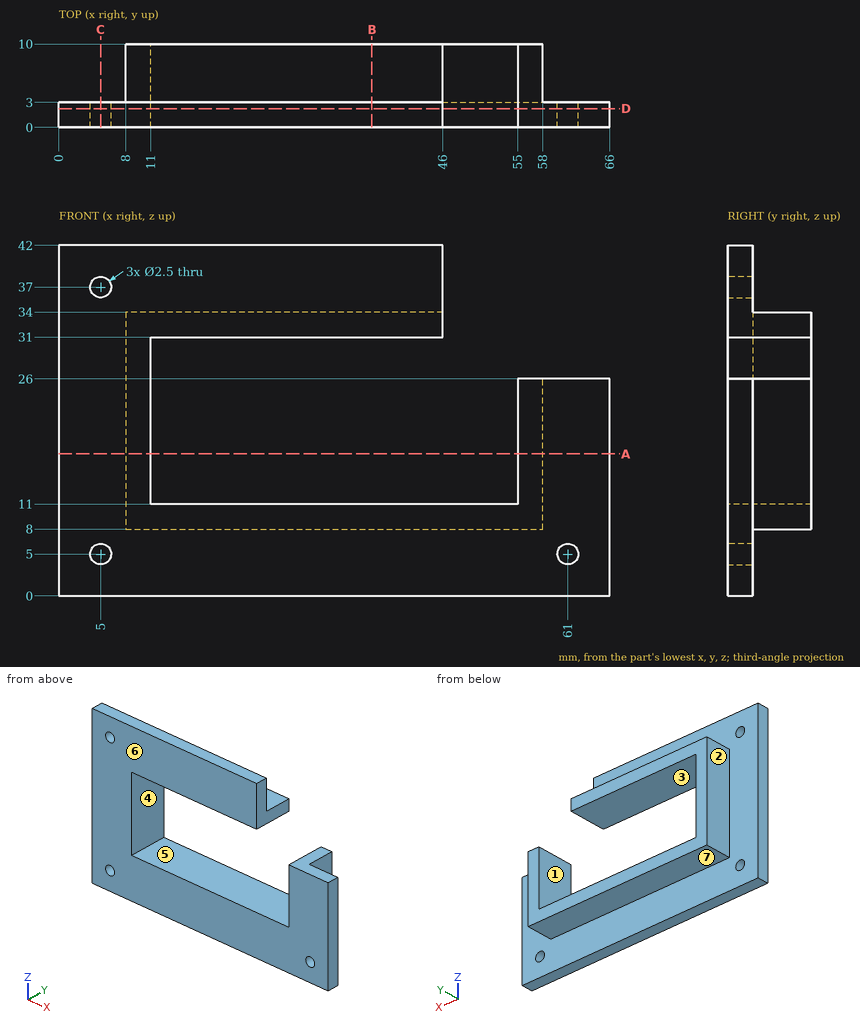
Job drawing, mm, ordinate dimensions from the low corner. One solid piece. A direction names the side the tool comes from. Round coordinates to 2 decimals unless told otherwise and drop trailing zeros. Loops run counter-clockwise (first coordinate to the right, second up) from the corner with the lowest first, then second, coordinate; pieces in that order, holes last. Notation, with made-up numbers: (46, 80) -> (105, 80) arc R28 cw to (105, 103) -> close; hole circle Ø7 at (-40, -12). An arc over 180 degrees is marked (long way). One line per item, written item: value. Start each with the question number.
Q1. Probe line 1 along X through (y, z) = (1.95, 5); line 2 along Z through (x, y) = (36.5, 2); line 3 along X through (y, z) = (1.65, 37). List the from-to ranges inside material, lowest first.
Q2. Cut at C-C on x = 5. List the corners of the cut face in (y, z).
Q3. 3-axis set-ups, long thin cutter, end or side, ignore diameter. For the marked faces 1, 2, 3 and 4: which of +Z, -Z, +X, -X, +Y, -Y reach the whole face in a straight line?
Q4. Cut at D-D on y = 2.25. List the corners of the cut face in (x, z).
Q5. Drop flat-ended pins along their axis: pin 1 Ø6 at (x, z) = (32.5, 28.5) entering from -Y; pin 2 Ø1 at (y, z) = (8.5, 26) entering from +X; pin 3 Ø4 at (x, z) = (5, 5) entering from +Y; pin 4 Ø3 at (x, y) = (51, 1) entering from +Z. Give the stop position or say it passes through.
Q6. Two-plate mould, pull along Z, no slides. Class the marked faces 5, 6 and 7: released by +Z, released by -Z, zero draft, split by the parting line, or undercut.
Q7. Cut at A-A on z = 17. List the corners of the cut face in (x, y), plus the area to 3 significant figures.
Q8. Cut at B-B on x = 37.5. List the corners of the cut face in (y, z), plus the area to 3 significant figures.
Computed:
1. line 1: 0 to 3.75, 6.25 to 59.75, 62.25 to 66
1. line 2: 0 to 11, 31 to 42
1. line 3: 0 to 3.75, 6.25 to 46
2. outline: (0, 0) -> (3, 0) -> (3, 3.75) -> (0, 3.75) -> close; (0, 6.25) -> (3, 6.25) -> (3, 35.75) -> (0, 35.75) -> close; (0, 38.25) -> (3, 38.25) -> (3, 42) -> (0, 42) -> close
3. face 1: +Z, +Y, -Y
3. face 2: +Z, -Z, -X, +Y
3. face 3: +X, +Y, -Y
3. face 4: +Y, -Y
4. outline: (0, 0) -> (66, 0) -> (66, 26) -> (55, 26) -> (55, 11) -> (11, 11) -> (11, 31) -> (46, 31) -> (46, 42) -> (0, 42) -> close; hole circle Ø2.5 at (5, 5); hole circle Ø2.5 at (5, 37); hole circle Ø2.5 at (61, 5)
5. pin 1: y = 0
5. pin 2: x = 58
5. pin 3: y = 3
5. pin 4: z = 11
6. face 5: undercut
6. face 6: zero draft
6. face 7: released by -Z
7. outline: (0, 0) -> (11, 0) -> (11, 10) -> (8, 10) -> (8, 3) -> (0, 3) -> close; (55, 0) -> (66, 0) -> (66, 3) -> (58, 3) -> (58, 10) -> (55, 10) -> close
7. area: 108 mm²
8. outline: (0, 0) -> (3, 0) -> (3, 8) -> (10, 8) -> (10, 11) -> (0, 11) -> close; (0, 31) -> (10, 31) -> (10, 34) -> (3, 34) -> (3, 42) -> (0, 42) -> close
8. area: 108 mm²
